Verification items for this drawing (mm, ordinates from the low corner). A direction names the side the tool comes from. Coordinates: 2 decimals unless noted, no trailing zeros. Order: outer loops, then holes, each group sorted by start corner. A loop starts at its lowest first (then second) coordinate and runs counter-clockwise, first axis right, second up. Notation, with made-up numbers: M -13,74 L -9,74 A22 cw -9,111 Z; hole C -25,23 d1. An arc over 180 degrees is marked long. Write item = value, one per line.
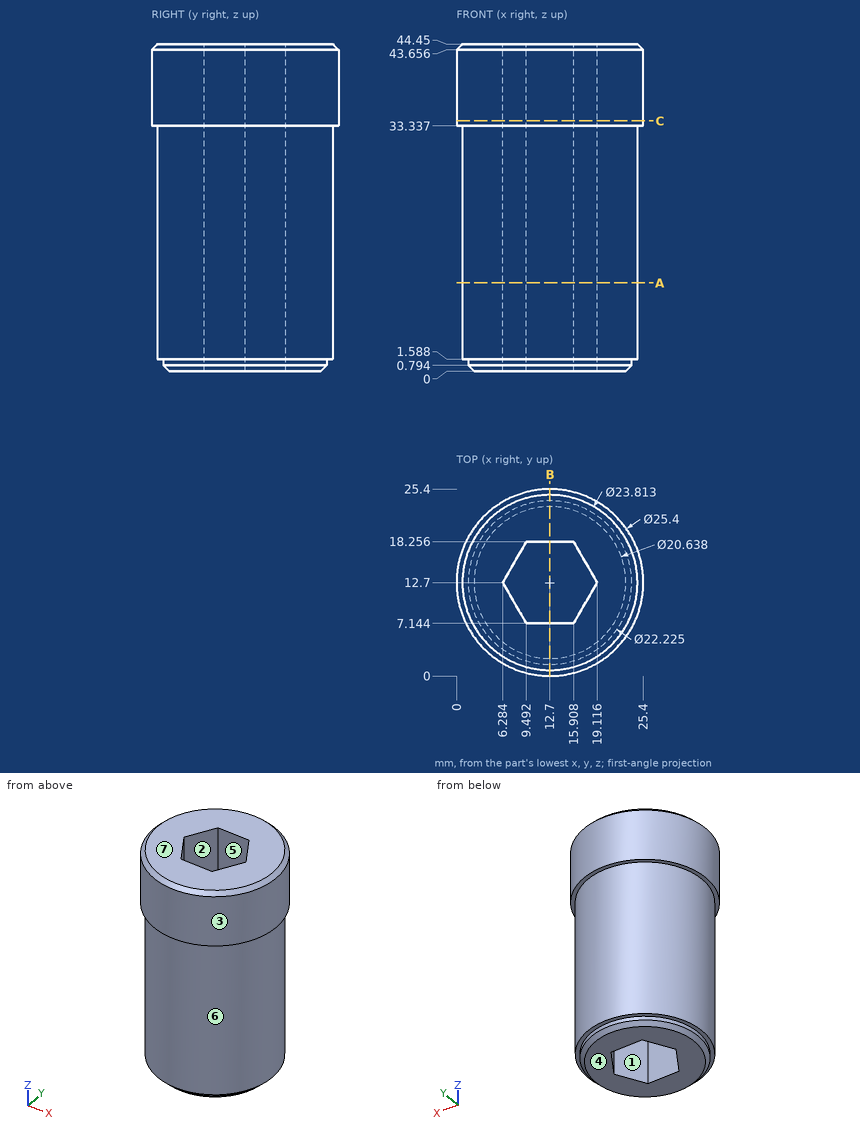
Item 1: Release check for a two-part mould opening along Y. For the marked faces 1, 2, 3 and 4 record: pulls with the +Y half, pulls with the -Y half, needs draft (parallel to the pull), parting line crosses it, or undercut.
Report:
face_1 = undercut
face_2 = undercut
face_3 = parting line crosses it
face_4 = needs draft
Item 2: Sectioned sample at A-A, the plane z = 12. Enter the section's corners in (x, y) (1 decimal).
Report:
outline = C 12.7,12.7 d23.8; hole M 6.3,12.7 L 9.5,7.1 L 15.9,7.1 L 19.1,12.7 L 15.9,18.3 L 9.5,18.3 Z
Item 3: Tool access check on the marked faces 5, 6 and 7. Record the directions out of +Z, -Z, +X, -X, +Y, -Y that give a thin tool (end or side, any length) a straight path to the whole face; none if there is none.
Report:
face_5 = +Z, -Z
face_6 = -Z
face_7 = +Z, +X, -X, +Y, -Y
Item 4: Sectioned sample at C-C, the plane z = 34. Enter the section's corners in (x, y) (1 decimal), then the cut area to 3 significant figures.
Report:
outline = C 12.7,12.7 d25.4; hole M 6.3,12.7 L 9.5,7.1 L 15.9,7.1 L 19.1,12.7 L 15.9,18.3 L 9.5,18.3 Z
area = 400 mm^2
Item 5: Sectioned sample at B-B, the plane x = 12.7. Enter the section's corners in (y, z).
Report:
outline = M 0,33.34 L 0.79,33.34 L 0.79,1.59 L 1.59,1.59 L 1.59,0.79 L 2.38,0 L 7.14,0 L 7.14,44.45 L 0.79,44.45 L 0,43.66 Z; M 18.26,0 L 23.02,0 L 23.81,0.79 L 23.81,1.59 L 24.61,1.59 L 24.61,33.34 L 25.4,33.34 L 25.4,43.66 L 24.61,44.45 L 18.26,44.45 Z
Item 6: Scan lines: L1, parallel to Y at x = 9.5, z = 31 (1 decimal); L2, parallel to Y at x = 10, z = 12 (1 decimal); L3, parallel to X at y = 16, z = 25.5. Record each from-to range of solid material in increasing order. Write a range as from..to.
Report:
L1 = 1.2..7.1, 18.3..24.2
L2 = 1.1..7.1, 18.3..24.3
L3 = 1.26..8.19, 17.21..24.14
Item 7: Gauge pin test, flat ends, axial feed: pin 1 (12 mm diameter, centred on x = 15, z = 9, fed in from +Y); pin 2 (12 mm diameter, centred on y = 16, z = 27, fed in from +X); pin 3 (2 mm diameter, centred on y = 8.5, z = 17, fed in from -X). Record the tip position at first contact, or that the pin passes through.
Report:
pin_1 = 24.61
pin_2 = 24.61
pin_3 = 1.23
